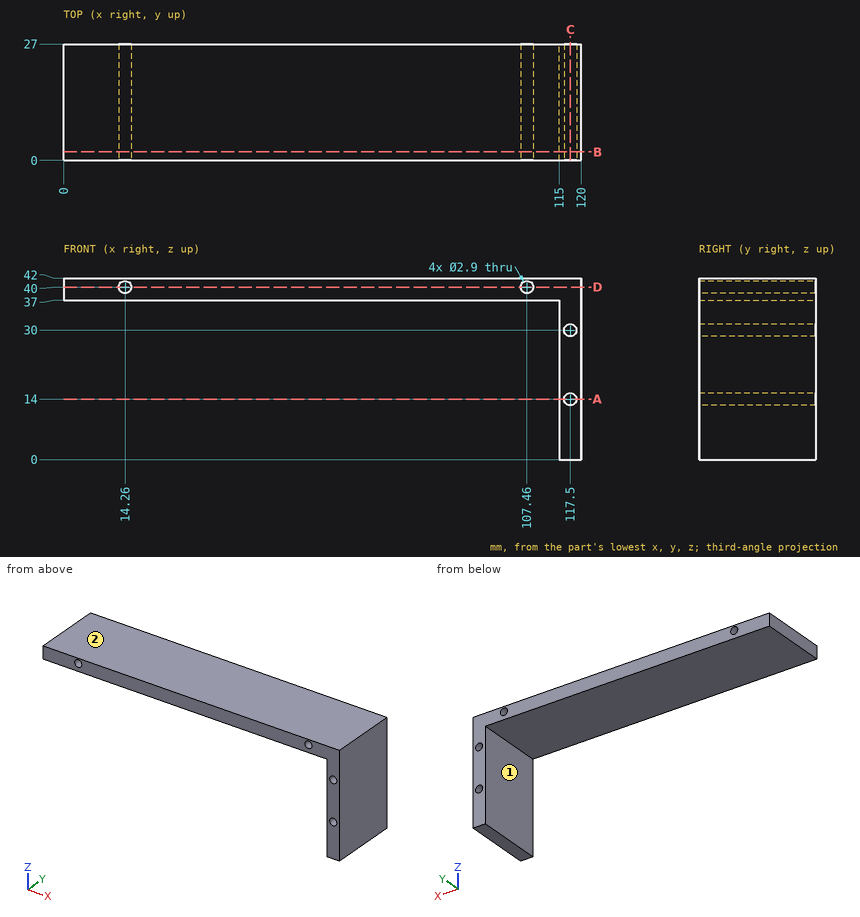
Source: three-view drawing plus pictorial views. Frame: mm from the lowest corner of the part. A direction names the side the tool comes from. Give positions to 0.01 mm unless a question says otherwise; leave off trailing zeros. Order: outer loops, then holes, each group sorted by start corner. A loop starts at its lowest first (then second) coordinate and runs counter-clockwise, first axis right, second up. Notation, with made-up numbers: M -38,53 L -17,53 A21 cw -17,86 Z; hole C 75.5,52.5 d3. An arc over 180 degrees is marked long. Return JSON: item names as keys, results as strings.
Item 1: First-contact query: P1, Ø3, axis at y = 23.5, z = 20.5, coming from the -X side; P2, Ø2.5, axis at x = 107.46, z = 40, coming from the -Y side; P3, Ø4, axis at x = 117.5, z = 30, coming from the -Y side; P4, Ø8, axis at x = 25.5, y = 10, coming from the -Z side. Flat tips, straight axial feed; report the tip coordinate or a pass-through.
Solutions:
{"P1": "x = 115", "P2": "through", "P3": "y = 0", "P4": "z = 37"}
Item 2: Cut plane D-D (z = 40). Return loops of the section in (x, y).
Solutions:
{"outline": "M 0,0 L 12.81,0 L 12.81,27 L 0,27 Z; M 15.71,0 L 106.01,0 L 106.01,27 L 15.71,27 Z; M 108.91,0 L 120,0 L 120,27 L 108.91,27 Z"}
Item 3: Cut plane C-C (x = 117.5). Return loops of the section in (y, z).
Solutions:
{"outline": "M 0,0 L 27,0 L 27,12.55 L 0,12.55 Z; M 0,15.45 L 27,15.45 L 27,28.55 L 0,28.55 Z; M 0,31.45 L 27,31.45 L 27,42 L 0,42 Z"}
Item 4: Access query for the marked faces 1 and 2. Directions: +Z, -Z, +X, -X, +Y, -Y. A direction counts if a zero-diameter tool reaches every point of the face in a straight line with its end or side. Return the directions, or none.
Solutions:
{"face 1": "-Z, -X, +Y, -Y", "face 2": "+Z, +X, -X, +Y, -Y"}
Item 5: Cut plane B-B (y = 2). Return loops of the section in (x, z).
Solutions:
{"outline": "M 0,37 L 115,37 L 115,0 L 120,0 L 120,42 L 0,42 Z; hole C 14.26,40 d2.9; hole C 107.46,40 d2.9; hole C 117.5,14 d2.9; hole C 117.5,30 d2.9"}
Item 6: Cut plane A-A (z = 14). Return loops of the section in (x, y), then the cut area to 3 significant figures.
Solutions:
{"outline": "M 115,0 L 116.05,0 L 116.05,27 L 115,27 Z; M 118.95,0 L 120,0 L 120,27 L 118.95,27 Z", "area": "56.7 mm^2"}
Item 7: Ray query, probe 1 along X at (y, z) = (18, 40); probe 2 along Z at (x, y) = (117.5, 15.5); probe 3 along X at (y, z) = (19.75, 30). Return the intervals inside material, ascending.
Solutions:
{"probe 1": "0 to 12.81, 15.71 to 106.01, 108.91 to 120", "probe 2": "0 to 12.55, 15.45 to 28.55, 31.45 to 42", "probe 3": "115 to 116.05, 118.95 to 120"}
